The model under review builds one solid part; all positions refer to its coordinate system, in mm. Round coordinates to 2 decimals unless told otherwise and drop trailing zeros. Loops run counter-clockwise (first coordinate to the right, second up) from the corner with the lowest first, then second, coordinate; pieces in that order, holes last. Notation, with made-up numbers: M 47,-20 L 105,-20 A7 cw 105,-15 Z; hole C 26,74.25 d10. An arc over 180 degrees is marked long. Return JSON: item names as keys, results as strings. Group by question number.
Q1. Consider section B-B (y = 3.5). State the section outline as (x, z) points, and give its area (3 significant figures).
Q2. Clearance check with a flat-ended pin moving along its axis: pin 1 Ø1.5 at (x, z) = (9.5, 0.5) entering from +Y (3 decimals). State where the tip first meets the part, or that it passes through.
Q3. Consider section D-D (x = 6). State the section outline as (y, z) points, and give its area (3 significant figures).
Q4. Consider section A-A (x = 0). State the section outline as (y, z) points, and give its area (3 significant figures).
Q5. To check wall thickness, follow line 1 along Y through (x, z) = (0, 3.6); line 2 along X through (y, z) = (3.25, 1.5); line 3 along X through (y, z) = (3.75, 4.5). State the ranges of each line that lie inside material, in increasing order.
Q6. Draft analysis for pull direction X (two halves, no side actions). For faces 1 (the face through (-13.07, 3.09, 3.04)), 2 (the face through (-0.521, 10.285, 2.958)), 3 (the face through (-0.04, 12.68, 3.04)), state which applies: pulls with the +X half, pulls with the -X half, needs draft (parallel to the pull), parting line crosses it, or undercut.
Q7. Consider section C-C (z = 1.75). State the section outline as (x, y) points.
from build123d import *

# Parameters (mm, degrees)
F1_DEPTH = 6
F2_R     = 4
F3_R     = 6
F4_R     = 4
F5_DEPTH = 6.001


with BuildPart() as f1:
    # F0 (on Top) → F1 (new body)
    with BuildSketch(Plane.XY):
        Polygon((0, 13.5), (-25, 0), (25, 0), align=None)
    extrude(amount=F1_DEPTH)

    # F2
    f2_edges = [f1.edges().sort_by_distance(p)[0] for p in [
        (25, 0, 3),
        (-25, 0, 3),
    ]]
    fillet(f2_edges, radius=F2_R)

    # F3
    f3_edges = [f1.edges().sort_by_distance(p)[0] for p in [
        (0, 13.5, 3),
    ]]
    fillet(f3_edges, radius=F3_R)

    # F4 (on Top) → F5 (cut, through all)
    with BuildSketch(Plane.XY):
        with Locations((0, 6.318788)):
            Circle(F4_R)
    extrude(amount=F5_DEPTH, mode=Mode.SUBTRACT)


solid = f1.part
Values:
{
 "1": {"outline": "M -13.14,0 L -2.84,0 L -2.84,6 L -13.14,6 Z; M 2.84,0 L 13.14,0 L 13.14,6 L 2.84,6 Z", "area": "124 mm2"},
 "2": {"pin 1": "stops at y = 8.775"},
 "3": {"outline": "M 0,0 L 10.26,0 L 10.26,6 L 0,6 Z", "area": "61.6 mm2"},
 "4": {"outline": "M 0,0 L 2.32,0 L 2.32,6 L 0,6 Z; M 10.32,0 L 12.68,0 L 12.68,6 L 10.32,6 Z", "area": "28.1 mm2"},
 "5": {"line 1": "y = 0 to 2.32, 10.32 to 12.68", "line 2": "x = -13.1 to -2.57, 2.57 to 13.1", "line 3": "x = -13.17 to -3.07, 3.07 to 13.17"},
 "6": {"face 1": "pulls with the -X half", "face 2": "undercut", "face 3": "parting line crosses it"},
 "7": {"outline": "M -11.07,7.52 A4 ccw -9.17,0 L 9.17,0 A4 ccw 11.07,7.52 L 2.85,11.96 A6 ccw -2.85,11.96 Z; hole C 0,6.32 d8"}
}
